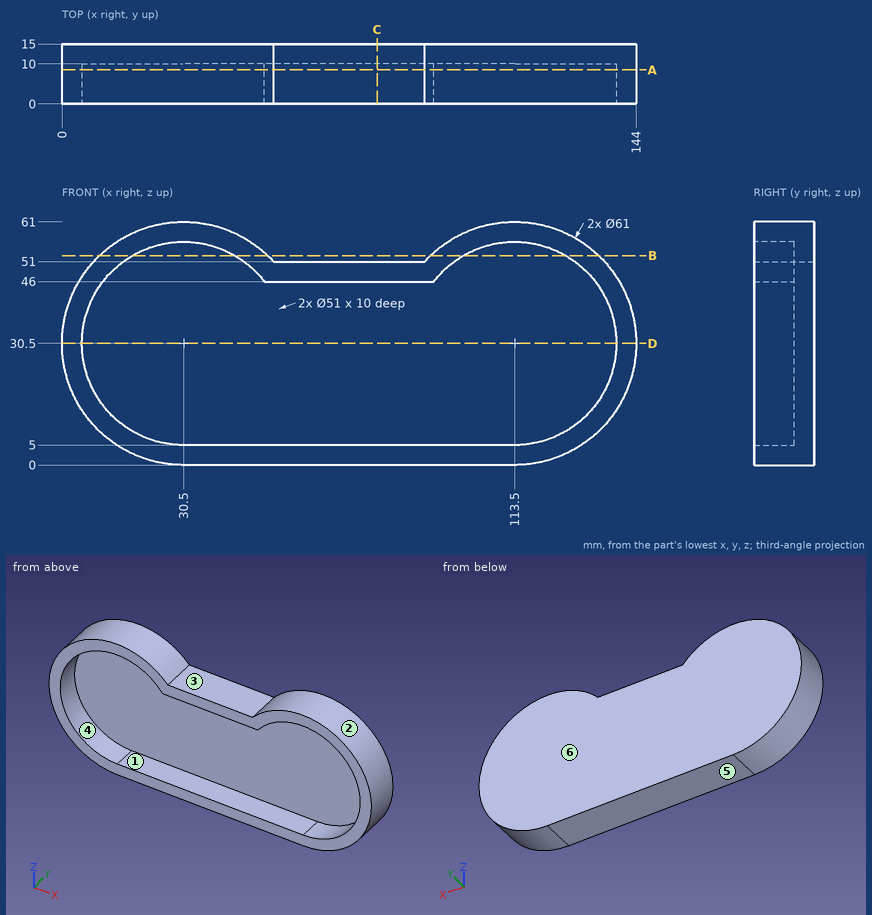
Geometry check sheet. Reference: drawing and pictorial views, mm from the part's lowest x, y, z. A direction names the side the tool comes from. Round coordinates to 2 decimals unless told otherwise and drop trailing zeros. Order: outer loops, then holes, each group sorted by start corner. A loop starts at its lowest first (then second) coordinate and runs counter-clockwise, first axis right, second up. Notation, with made-up numbers: M 46.25,36 L 99.25,36 A27 ccw 99.25,63 Z; hole C 22.5,81 d2. An arc over 180 degrees is marked long. Write item = value, one per line.
Q1. Release check for a two-part mould opening along Z. For the marked faces 4, 5 and 6 record: released by +Z, released by -Z, zero draft, split by the parting line, or undercut.
Answer block:
face_4 = undercut
face_5 = released by -Z
face_6 = zero draft
Q2. Scan lines: line 1 (X direction, y = 4.75, z = 30.5); line 2 (Z direction, x = 59, y = 5.75); line 3 (Z direction, x = 51, y = 8.5). Record each from-to range of solid material in increasing order.
Answer block:
line_1 = 0 to 5, 139 to 144
line_2 = 0 to 5, 46 to 51
line_3 = 0 to 5, 46 to 53.08
Q3. Section check C-C (x = 79). Enter the section's corners in (y, z), plus the area to 3 significant figures.
Answer block:
outline = M 0,0 L 15,0 L 15,51 L 0,51 L 0,46 L 10,46 L 10,5 L 0,5 Z
area = 355 mm^2
Q4. Section check D-D (z = 30.5). Enter the section's corners in (x, y).
Answer block:
outline = M 0,0 L 5,0 L 5,10 L 139,10 L 139,0 L 144,0 L 144,15 L 0,15 Z
Q5. Depth check by flat-ended pin: pin 1 Ø1.5 at (x, y) = (25.5, 2.5) entering from +Z; pin 2 Ø8 at (x, y) = (126, 9) entering from +Z; pin 3 Ø1.5 at (y, z) = (11, 36) entering from -X; pin 4 Ø3 at (x, y) = (78.5, 3.5) entering from -Z. Enter the tip coordinate at first touch or a pass-through.
Answer block:
pin_1 = 60.7
pin_2 = 59.79
pin_3 = 0.37
pin_4 = 0
Q6. Section check B-B (z = 52.5). Enter the section's corners in (x, y).
Answer block:
outline = M 9.38,0 L 17.61,0 L 17.61,10 L 43.39,10 L 43.39,0 L 51.62,0 L 51.62,15 L 9.38,15 Z; M 92.38,0 L 100.61,0 L 100.61,10 L 126.39,10 L 126.39,0 L 134.62,0 L 134.62,15 L 92.38,15 Z
Q7. Set-up check for the marked faces 1, 2 and 3: record each of +Z, -Z, +X, -X, +Y, -Y from which the full face is reachable in a straight line by a thin tool's end or side.
Answer block:
face_1 = -Y
face_2 = +Y, -Y
face_3 = +Z, +Y, -Y
Q8. Section check A-A (y = 8.5). Enter the section's corners in (x, z).
Answer block:
outline = M 30.5,0 L 113.5,0 A30.5 ccw long 90.92,51 L 53.08,51 A30.5 ccw long Z; hole M 30.5,5 L 113.5,5 A25.5 ccw long 93.25,46 L 50.75,46 A25.5 ccw long Z
